Part model, mm, in its own coordinate system. Face numbers are marked on the shaded views. A direction names the side the tool comes from. Round coordinates to 2 decimals unless told otherwise and drop trailing zeros. Write each loop counter-clockwise with the first axis right and the second up, starting at its lowest first coordinate (ties: lowest second). Pieces come first, ordered by that corner, then holes.
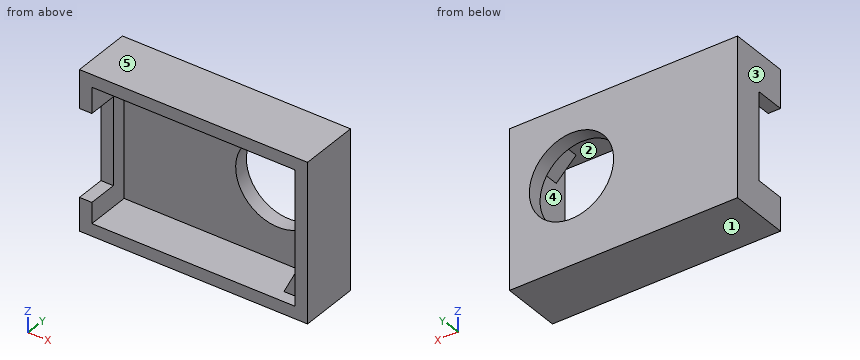
```python
from build123d import *

# Parameters (mm, degrees)
SKETCH2_W           = 40
SKETCH2_H           = 26
BOSS_EXTRUDE1_DEPTH = 3
SKETCH3_R           = 8.5
CUT_EXTRUDE1_DEPTH  = 3
SKETCH4_W           = 26
SKETCH4_H           = 3
BOSS_EXTRUDE2_DEPTH = 3
SKETCH5_W           = 26
SKETCH5_H           = 3
BOSS_EXTRUDE3_DEPTH = 3
SKETCH6_W           = 46
SKETCH6_H           = 3
BOSS_EXTRUDE4_DEPTH = 3
SKETCH7_W           = 46
SKETCH7_H           = 3
BOSS_EXTRUDE5_DEPTH = 3
SKETCH8_W           = 41
SKETCH8_H           = 27
BOSS_EXTRUDE6_DEPTH = 9
BOSS_EXTRUDE7_DEPTH = 6.6
SKETCH10_W          = 17.601141336
SKETCH10_H          = 6
CUT_EXTRUDE2_DEPTH  = 6.6


with BuildPart() as part:
    # Sketch2 → Boss-Extrude1 (new body)
    with BuildSketch(Plane(origin=(0, 0, 0), x_dir=(1, 0, 0), z_dir=(0, 1, 0))):
        Rectangle(SKETCH2_W, SKETCH2_H)
    extrude(amount=BOSS_EXTRUDE1_DEPTH)

    # Sketch3 → Cut-Extrude1 (cut)
    with BuildSketch(Plane(origin=(0, 3, 0), x_dir=(1, 0, 0), z_dir=(0, 1, 0))):
        with Locations(Location((10.5, -1.7, 0), (0, 0, 270))):
            Circle(SKETCH3_R)
    extrude(amount=-CUT_EXTRUDE1_DEPTH, mode=Mode.SUBTRACT)

    # Sketch4 → Boss-Extrude2 (add)
    with BuildSketch(Plane(origin=(20, 0, 0), x_dir=(0, 0, -1), z_dir=(1, 0, 0))):
        with Locations((0, 1.5)):
            Rectangle(SKETCH4_W, SKETCH4_H)
    extrude(amount=BOSS_EXTRUDE2_DEPTH)

    # Sketch5 → Boss-Extrude3 (add)
    with BuildSketch(Plane.ZY.offset(20)):
        with Locations((0, 1.5)):
            Rectangle(SKETCH5_W, SKETCH5_H)
    extrude(amount=BOSS_EXTRUDE3_DEPTH)

    # Sketch6 → Boss-Extrude4 (add)
    with BuildSketch(Plane.XY.offset(13)):
        with Locations((0, 1.5)):
            Rectangle(SKETCH6_W, SKETCH6_H)
    extrude(amount=BOSS_EXTRUDE4_DEPTH)

    # Sketch7 → Boss-Extrude5 (add)
    with BuildSketch(Plane(origin=(0, 0, -13), x_dir=(-1, 0, 0), z_dir=(0, 0, -1))):
        with Locations((0, 1.5)):
            Rectangle(SKETCH7_W, SKETCH7_H)
    extrude(amount=BOSS_EXTRUDE5_DEPTH)

    # Sketch8 → Boss-Extrude6 (add)
    with BuildSketch(Plane.XZ):
        Polygon((23, 13), (23, 16), (20, 16), (-20, 16), (-23, 16), (-23, 13), (-23, -13), (-23, -16), (-20, -16), (20, -16), (23, -16), (23, -13), align=None)
        Rectangle(SKETCH8_W, SKETCH8_H, mode=Mode.SUBTRACT)
    extrude(amount=BOSS_EXTRUDE6_DEPTH)

    # Sketch9 → Boss-Extrude7 (add)
    with BuildSketch(Plane.XZ):
        Polygon((20.5, 9.5), (16.5, 13.5), (20.5, 13.5), align=None)
        Polygon((20.5, -5.5), (16.5, -13.5), (20.5, -13.5), align=None)
    extrude(amount=BOSS_EXTRUDE7_DEPTH)

    # Sketch10 → Cut-Extrude2 (cut)
    with BuildSketch(Plane.ZY.offset(23)):
        with Locations((-0.508683185, -6)):
            Rectangle(SKETCH10_W, SKETCH10_H)
    extrude(amount=-CUT_EXTRUDE2_DEPTH, mode=Mode.SUBTRACT)


solid = part.part
```
Q1. Cut at D-D on x = -8. Write the cut outline in (y, z), plus the area to 3 significant figures.
Values follow:
outline: (-9, -16) - (3, -16) - (3, 16) - (-9, 16) - (-9, 13.5) - (0, 13.5) - (0, -13.5) - (-9, -13.5) - close
area: 141 mm2
Q2. Cut at A-A on z = 1.7. Write the cut outline in (x, y), plus the area to 3 significant figures.
Values follow:
outline: (-23, -3) - (-20.5, -3) - (-20.5, 0) - (2, 0) - (2, 3) - (-23, 3) - close; (19, 0) - (20.5, 0) - (20.5, -9) - (23, -9) - (23, 3) - (19, 3) - close
area: 117 mm2
Q3. Wall check: L1, parallel to Z at x = 2.5, y = -4.5; L2, parallel to X at y = 1.85, z = 1.7; L3, parallel to X at y = -1.75, z = 9. Give the ranges that are in metal, low to high.
Values follow:
L1: z = -16 to -13.5, 13.5 to 16
L2: x = -23 to 2, 19 to 23
L3: x = -23 to -20.5, 20.5 to 23
Q4. Drop flat-ended pins along their axis: pin 1 (4.5 mm diameter, centred on x = 18.5, z = -11, fed in from -Y); pin 2 (2 mm diameter, centred on x = -22, z = 2.5, fed in from -Y). Give the stop position or say it passes through.
Values follow:
pin 1: stops at y = -9
pin 2: stops at y = -3
Q5. Mould opens along Z. For the marked faces 3, 4 and 5 say: +Z half, -Z half, draft (parallel to the pull), parting line (faces both ways), or undercut.
Values follow:
face 3: draft
face 4: undercut
face 5: +Z half
Q6. Cut at C-C on y = -7.5. Write the cut outline in (x, z), plus the area to 3 significant figures.
Values follow:
outline: (-23, -16) - (23, -16) - (23, 16) - (-23, 16) - (-23, 8.29) - (-20.5, 8.29) - (-20.5, 13.5) - (20.5, 13.5) - (20.5, -13.5) - (-20.5, -13.5) - (-20.5, -9.31) - (-23, -9.31) - close
area: 321 mm2
Q7. Which spindle directions (+Z, -Z, +X, -X, +Y, -Y) get a long thin tool onto all of the face, cutting with end or side? Do the marked faces 1 and 2. Say none if no direction does.
Values follow:
face 1: -Z, +X, -X, +Y, -Y
face 2: -Y
Q8. Cut at B-B on x = 10.5. Write the cut outline in (y, z).
Values follow:
outline: (-9, -16) - (3, -16) - (3, -6.8) - (0, -6.8) - (0, -13.5) - (-9, -13.5) - close; (-9, 13.5) - (0, 13.5) - (0, 10.2) - (3, 10.2) - (3, 16) - (-9, 16) - close
